Here's how the part is built. I have some questions about the finished solid (model axes, mm). A direction names the side the tool comes from. Coordinates: 2 decimals unless noted, no trailing zeros. Write each loop counter-clockwise with the first axis right and the second up, starting at its lowest first coordinate (ties: lowest second). Pieces come first, ordered by that corner, then holes.
(1) Imagine slicing it at C-C, the plane y = 391.5. List the corners of the cut face in (x, z) for me, plus the area to 3 significant figures.
(2) For pin 1 Ø3 at (x, z) = (7.5, 140) entering from -Y; pin 2 Ø2 at (x, z) = (4.5, 80) entering from -Y; pin 3 Ø2 at (x, y) = (10, 232.5) entering from +Z, each with a flat end and sliding along its axis, tell me the tip position at first contact or that it passes through.
(3) Thinking about a two-plate mould opening in Z: for faces 3 (the flat face through (1.476, 230, 133)), 4 (the flat face through (6, 256, 0)), 5 (the flat face through (7, 251, 6.5)), 6 (the flat face through (7, 492.371, 142)), which applies, released by +Z, released by -Z, zero draft, split by the parting line, or undercut?
(4) Please list where these lines run through material, in increasing order: probe 1 along Z at (x, y) = (8.25, 179.5); probe 2 along Y at (x, z) = (7.25, 257.5); probe 3 along Y at (x, z) = (5.5, 127).
(5) Which directions (+Z, -Z, +X, -X, +Y, -Y) give clear straight access to the entire face, cutting with the end or side of a thin tool? Please do faces 1 (the flat face through (6.406, 250.871, 146.016)), 2 (the flat face through (6.546, 258.013, 145.925)).
(6) Imagine slicing it at A-A, the plane x = 7. List the corners of the cut face in (y, z) for me.
(7) Imagine slicing it at B-B, the plane z = 113.5. List the corners of the cut face in (x, y) for me.
```python
from build123d import *

# Parameters (mm, degrees)
F0_W     = 10
F0_H     = 500
F1_DEPTH = 288
F3_DEPTH = 10
F5_DEPTH = 10
F6_W     = 10
F6_H     = 10
F7_DEPTH = 1


with BuildPart() as f1:
    # F0 (on Top) → F1 (new body)
    with BuildSketch(Plane.XY):
        with Locations((6.476007, 247.370639)):
            Rectangle(F0_W, F0_H)
    extrude(amount=F1_DEPTH)

    # F2 (on face) → F3 (cut)
    with BuildSketch(Plane(origin=(1.476007, 0, 0), x_dir=(0, -1, 0), z_dir=(-1, 0, 0))):
        Polygon((2.629361, 288), (-497.370639, 288), (2.629361, 0), align=None)
    extrude(amount=-F3_DEPTH, mode=Mode.SUBTRACT)

    # F4 (on face) → F5 (cut)
    with BuildSketch(Plane.YZ.offset(11.476007)):
        Polygon((492.370639, 281.5), (17, 6.5), (492.370639, 6.5), align=None)
    extrude(amount=-F5_DEPTH, mode=Mode.SUBTRACT)

    # F6 (on face) → F7 (join)
    with BuildSketch(Plane(origin=(0, 0, 0), x_dir=(1, 0, 0), z_dir=(0, 0, -1))):
        with Locations((6.476007, -2.370639)):
            Rectangle(F6_W, F6_H)
    extrude(amount=F7_DEPTH)


solid = f1.part
```
Recorded:
1. outline: (1.48, 0) - (11.48, 0) - (11.48, 6.5) - (1.48, 6.5) - close; (1.48, 223.15) - (11.48, 223.15) - (11.48, 227.02) - (1.48, 227.02) - close
1. area: 104 mm2
2. pin 1: stops at y = 237.82
2. pin 2: stops at y = 134.52
2. pin 3: stops at z = 136.01
3. face 3: zero draft
3. face 4: released by -Z
3. face 5: undercut
3. face 6: undercut
4. probe 1: z = 0 to 6.5, 100.51 to 104.91
4. probe 2: y = 444.42 to 450.88, 492.37 to 497.37
4. probe 3: y = 217.86 to 225.3, 492.37 to 497.37
5. face 1: +Z, +X, -X, -Y
5. face 2: +X, -X
6. outline: (-2.63, -1) - (7.37, -1) - (7.37, 0) - (497.37, 0) - (497.37, 288) - (-2.63, 0) - close; hole (17, 6.5) - (492.37, 6.5) - (492.37, 281.5) - close
7. outline: (1.48, 194.42) - (11.48, 194.42) - (11.48, 201.96) - (1.48, 201.96) - close; (1.48, 492.37) - (11.48, 492.37) - (11.48, 497.37) - (1.48, 497.37) - close
